Geometry check sheet. Reference: the model listing, model coordinates, mm. Face numbers are marked on the shaded views. A direction names the side the tool comes from. Round coordinates to 2 decimals unless told otherwise and drop trailing zeros. Order: outer loops, then holes, each group sorted by start corner. A loop starts at its lowest first (then second) coordinate and runs counter-clockwise, first axis right, second up.
```python
from build123d import *

# Parameters (mm, degrees)
F0_W      = 50
F0_H      = 40
F1_DEPTH  = 3
F2_W      = 3
F2_H      = 40
F3_DEPTH  = 50
F4_W      = 40
F4_H      = 3
F5_DEPTH  = 10
F6_W      = 40
F6_H      = 3
F7_DEPTH  = 10
F9_D      = 3
F8_R      = 12
F10_DEPTH = 25
F12_D     = 3
F14_D     = 3


with BuildPart() as f1:
    # F0 (on Top) → F1 (new body)
    with BuildSketch(Plane.XY):
        Rectangle(F0_W, F0_H)
    extrude(amount=F1_DEPTH)

    # F2 (on face) → F3 (join)
    with BuildSketch(Plane.XY.offset(3)):
        with Locations((23.5, 0)):
            Rectangle(F2_W, F2_H)
        with Locations((-23.5, 0)):
            Rectangle(F2_W, F2_H)
    extrude(amount=F3_DEPTH)

    # F4 (on face) → F5 (join)
    with BuildSketch(Plane.YZ.offset(25)):
        with Locations((0, 51.5)):
            Rectangle(F4_W, F4_H)
    extrude(amount=F5_DEPTH)

    # F6 (on face) → F7 (join)
    with BuildSketch(Plane(origin=(-25, 0, 0), x_dir=(0, -1, 0), z_dir=(-1, 0, 0))):
        with Locations((0, 51.5)):
            Rectangle(F6_W, F6_H)
    extrude(amount=F7_DEPTH)

    # F9 (through all)
    with Locations(Plane(origin=(0, 0, 0), x_dir=(1, 0, 0), z_dir=(0, 0, -1))):
        with Locations((-15.5, 15.5), (15.5, 15.5), (15.5, -15.5), (-15.5, -15.5)):
            Hole(F9_D / 2)

    # F8 (on face) → F10 (cut)
    with BuildSketch(Plane(origin=(0, 0, 0), x_dir=(1, 0, 0), z_dir=(0, 0, -1))):
        Circle(F8_R)
    extrude(amount=-F10_DEPTH, mode=Mode.SUBTRACT)

    # F12 (through all)
    with Locations(Plane.XY.offset(53)):
        with Locations((-28.5, -10), (-28.5, 10)):
            Hole(F12_D / 2)

    # F14 (through all)
    with Locations(Plane.XY.offset(53)):
        with Locations((28.5, 10), (28.5, -10)):
            Hole(F14_D / 2)


solid = f1.part
```
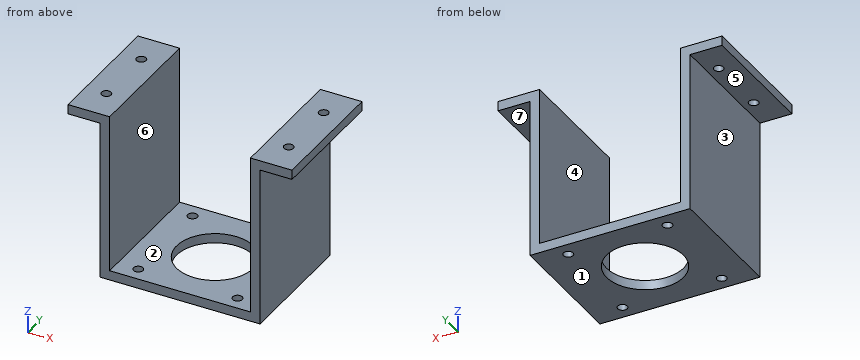
(1) Sectioned sample at A-A, the plane x = -28.5. Record the cut outline in (y, z).
Returned:
outline: (-20, 50) - (-11.5, 50) - (-11.5, 53) - (-20, 53) - close; (-8.5, 50) - (8.5, 50) - (8.5, 53) - (-8.5, 53) - close; (11.5, 50) - (20, 50) - (20, 53) - (11.5, 53) - close
(2) Sectioned sample at B-B, the plane z = 47. Record the cut outline in (x, y), and give its area (3 significant figures).
Returned:
outline: (-25, -20) - (-22, -20) - (-22, 20) - (-25, 20) - close; (22, -20) - (25, -20) - (25, 20) - (22, 20) - close
area: 240 mm2
(3) Draft check along X on the marked faces 1, 2, 3 and 4. Enter one of: released by +X, released by -X, zero draft, split by the parting line, or undercut.
Returned:
face 1: zero draft
face 2: undercut
face 3: released by -X
face 4: undercut
(4) Sectioned sample at D-D, the plane x = -10.5. Record the cut outline in (y, z).
Returned:
outline: (-20, 0) - (-5.81, 0) - (-5.81, 3) - (-20, 3) - close; (5.81, 0) - (20, 0) - (20, 3) - (5.81, 3) - close
(5) Material ranges on line 1 (Y direction, x = 28.5, z = 51.25); line 2 (Y direction, x = -15.5, z = 0.6); line 3 (X direction, y = 1, z = 29), recorded low to high.
Returned:
line 1: y = -20 to -11.5, -8.5 to 8.5, 11.5 to 20
line 2: y = -20 to -17, -14 to 14, 17 to 20
line 3: x = -25 to -22, 22 to 25
(6) Sectioned sample at C-C, the plane y = -15.5. Record the cut outline in (x, z), and give its area (3 significant figures).
Returned:
outline: (-35, 50) - (-25, 50) - (-25, 0) - (-17, 0) - (-17, 3) - (-22, 3) - (-22, 53) - (-35, 53) - close; (-14, 0) - (14, 0) - (14, 3) - (-14, 3) - close; (17, 0) - (25, 0) - (25, 50) - (35, 50) - (35, 53) - (22, 53) - (22, 3) - (17, 3) - close
area: 492 mm2
(7) Set-up check for the marked faces 5, 6 and 7: record each of +Z, -Z, +X, -X, +Y, -Y from which the full face is reachable in a straight line by a thin tool's end or side.
Returned:
face 5: -Z, -X, +Y, -Y
face 6: +Z, +Y, -Y
face 7: -Z, +X, +Y, -Y
(8) Depth check by flat-ended pin: P1, Ø5, axis at x = 29.5, y = -5.5, coming from the -Z side; P2, Ø1.5, axis at x = -13.5, y = -8.5, coming from the +Z side; P3, Ø6, axis at y = -4, z = 19.5, coming from the +X side. Enter the tip coordinate at first touch or a pass-through.
Returned:
P1: stops at z = 50
P2: stops at z = 3
P3: stops at x = 25
